Verification items for the finished model (mm, model axes). A direction names the side the tool comes from. Give positions to 0.01 mm unless a question says otherwise; leave off trailing zeros. Order: outer loops, then holes, each group sorted by start corner. A loop starts at its lowest first (then second) coordinate and runs counter-clockwise, first axis right, second up. Notation, with made-up numbers: (-37, -24.75) - (1, -24.75) arc R30 cw to (1, 10.25) - close; hole circle Ø8 at (1.5, -32.75). An arc over 180 degrees is marked (long way). Answer as a JSON object with one key per item and string values. Group by question number.
(1) Mould release check, pull along X, two halves, no side actions. Record for faces 1 (the face through (15, -8, 272)), 2 (the face through (7, 0, 272)), 3 (the face through (14, -8, 272)): +X half, -X half, draft (parallel to the pull), parting line (faces both ways), or undercut.
(2) Thickness scan on line 1 (X direction, y = -14.7, z = 158); line 2 (Y direction, x = 6, z = 250.5); line 3 (X direction, y = -5.75, z = 372.5). Record the ranges inside material, lowest first.
(3) Access from +Z, -Z, +X, -X, +Y, -Y to the whole of each face (thin tool, end or side, straight path). Record for faces 4 (the face through (0.7, -7.4, 0)), 5 (the face through (1, -8, 272)).
(4) Depth check by flat-ended pin: pin 1 Ø2.5 at (x, z) = (10.5, 546) entering from +Y. Enter the tip coordinate at first touch or a pass-through.
(5) Section check B-B (y = -6.5). Record the boundary of the cut face in (x, z).
(6) Section check A-A (z = 296). Record the boundary of the cut face in (x, y), then the cut area to 3 significant figures.
```python
from build123d import *

# Parameters (mm, degrees)
SKETCH_1_W          = 15
SKETCH_1_H          = 15
SKETCH_1_W_2        = 13
SKETCH_1_H_2        = 13
EXTRUDE_1_DEPTH     = 551
SKETCH_2_R          = 1.6
SKETCH_2_R_2        = 2.6
CUT_EXTRUDE_1_DEPTH = 552.408197255


with BuildPart() as part:
    # 草图1 → 拉伸-薄壁1 (new body)
    with BuildSketch(Plane.XY):
        with Locations((7.5, -7.5)):
            Rectangle(SKETCH_1_W, SKETCH_1_H)
        with Locations((7.5, -7.5)):
            Rectangle(SKETCH_1_W_2, SKETCH_1_H_2, mode=Mode.SUBTRACT)
    extrude(amount=EXTRUDE_1_DEPTH)

    # 草图2 → 切除-拉伸1 (cut, through all)
    with BuildSketch(Plane(origin=(0, 0, 0), x_dir=(1, 0, 0), z_dir=(0, 1, 0))):
        with Locations(Location((4.5, -5, 0), (0, 0, 270))):
            Circle(SKETCH_2_R)
        with Locations(Location((10.5, -5, 0), (0, 0, 90))):
            Circle(SKETCH_2_R)
        with Locations(Location((10.5, -11, 0), (0, 0, 270))):
            Circle(SKETCH_2_R)
        with Locations(Location((4.5, -11, 0), (0, 0, 90))):
            Circle(SKETCH_2_R)
        with Locations(Location((4.5, -540, 0), (0, 0, 270))):
            Circle(SKETCH_2_R)
        with Locations(Location((10.5, -540, 0), (0, 0, 90))):
            Circle(SKETCH_2_R)
        with Locations(Location((10.5, -546, 0), (0, 0, 270))):
            Circle(SKETCH_2_R)
        with Locations(Location((4.5, -546, 0), (0, 0, 90))):
            Circle(SKETCH_2_R)
        with Locations(Location((4.75, -80, 0), (0, 0, 270))):
            Circle(SKETCH_2_R_2)
        with Locations(Location((4.5, -152, 0), (0, 0, 270))):
            Circle(SKETCH_2_R)
        with Locations(Location((10.5, -152, 0), (0, 0, 90))):
            Circle(SKETCH_2_R)
        with Locations(Location((10.5, -158, 0), (0, 0, 270))):
            Circle(SKETCH_2_R)
        with Locations(Location((4.5, -158, 0), (0, 0, 90))):
            Circle(SKETCH_2_R)
        with Locations(Location((4.75, -471, 0), (0, 0, 90))):
            Circle(SKETCH_2_R_2)
        with Locations(Location((4.5, -393, 0), (0, 0, 270))):
            Circle(SKETCH_2_R)
        with Locations(Location((10.5, -393, 0), (0, 0, 90))):
            Circle(SKETCH_2_R)
        with Locations(Location((10.5, -399, 0), (0, 0, 270))):
            Circle(SKETCH_2_R)
        with Locations(Location((4.5, -399, 0), (0, 0, 90))):
            Circle(SKETCH_2_R)
    extrude(amount=-CUT_EXTRUDE_1_DEPTH, mode=Mode.SUBTRACT)


solid = part.part
```
Solutions:
{
 "1": {"face 1": "+X half", "face 2": "draft", "face 3": "undercut"},
 "2": {"line 1": "x = 0 to 2.9, 6.1 to 8.9, 12.1 to 15", "line 2": "y = -15 to -14, -1 to 0", "line 3": "x = 0 to 1, 14 to 15"},
 "3": {"face 4": "-Z, +X, -X, +Y, -Y", "face 5": "+Z, -Z"},
 "4": {"pin 1": "passes through"},
 "5": {"outline": "(0, 0) - (1, 0) - (1, 551) - (0, 551) - close; (14, 0) - (15, 0) - (15, 551) - (14, 551) - close"},
 "6": {"outline": "(0, -15) - (15, -15) - (15, 0) - (0, 0) - close; hole (1, -14) - (14, -14) - (14, -1) - (1, -1) - close", "area": "56.0 mm2"}
}
